Design review of the part built by this model. Coordinates are the model's own, in mm. A direction names the side the tool comes from. Give positions to 0.01 mm unless a question says otherwise; leave off trailing zeros. Loops run counter-clockwise (first coordinate to the right, second up) from the corner with the lowest first, then second, coordinate; pieces in that order, holes last. Notation, with made-up numbers: M -2,6.25 L 55,6.25 A15 ccw 55,13.25 Z; hole C 64,-24.5 d1. An arc over 180 degrees is marked long. Answer as CSV lines item,"result".
```python
from build123d import *

# Parameters (mm, degrees)
SKETCH_1_R          = 5.5
EXTRUDE_1_DEPTH     = 2
SKETCH_2_R          = 3.5
EXTRUDE_2_DEPTH     = 4.5
SKETCH_3_R          = 2
CUT_EXTRUDE_1_DEPTH = 5
CHAMFER_1_SIZE      = 0.5
FILLET_1_R          = 0.2


with BuildPart() as part:
    # 草图1 → 凸台-拉伸1 (new body)
    with BuildSketch(Plane(origin=(0, 0, 0), x_dir=(1, 0, 0), z_dir=(0, 1, 0))):
        with Locations(Location((0, 0, 0), (0, 0, 270))):
            Circle(SKETCH_1_R)
    extrude(amount=EXTRUDE_1_DEPTH)

    # 草图2 → 凸台-拉伸2 (add)
    with BuildSketch(Plane(origin=(0, 2, 0), x_dir=(1, 0, 0), z_dir=(0, 1, 0))):
        with Locations(Location((0, 0, 0), (0, 0, 270))):
            Circle(SKETCH_2_R)
    extrude(amount=EXTRUDE_2_DEPTH)

    # 草图3 → 切除-拉伸1 (cut)
    with BuildSketch(Plane(origin=(0, 6.5, 0), x_dir=(1, 0, 0), z_dir=(0, 1, 0))):
        with Locations(Location((0, 0, 0), (0, 0, 270))):
            Circle(SKETCH_3_R)
    extrude(amount=-CUT_EXTRUDE_1_DEPTH, mode=Mode.SUBTRACT)

    # 倒角1
    chamfer_1_edges = [part.edges().sort_by_distance(p)[0] for p in [
        (0, 0, -5.5),
    ]]
    chamfer(chamfer_1_edges, length=CHAMFER_1_SIZE)

    # 圆角1
    fillet_1_edges = [part.edges().sort_by_distance(p)[0] for p in [
        (0, 6.5, -3.5),
    ]]
    fillet(fillet_1_edges, radius=FILLET_1_R)


solid = part.part
```
1. For P1, Ø3, axis at x = 3, y = 4, coming from the -Z side; P2, Ø2, axis at y = 4, z = 2.5, coming from the -X side; P3, Ø3, axis at x = -3.5, z = 1.5, coming from the +Y side; P4, Ø1.5, axis at x = 3.5, y = 1, coming from the -Z side, all flat-tipped, find the tip position at first contact; note any pin that passes through.
Answer block:
P1,"z = -3.16"
P2,"x = -3.16"
P3,"y = 6.5"
P4,"z = -4.76"
2. We need section A-A, the plane x = 0. Write out the cut boundary in (y, z), plus the area to 3 significant figures.
Answer block:
outline,"M 0,-5 L 0.5,-5.5 L 2,-5.5 L 2,-3.5 L 6.3,-3.5 A0.2 ccw 6.5,-3.3 L 6.5,-2 L 1.5,-2 L 1.5,2 L 6.5,2 L 6.5,3.3 A0.2 ccw 6.3,3.5 L 2,3.5 L 2,5.5 L 0.5,5.5 L 0,5 Z"
area,"33.2 mm²"
3. For faces 4 (the flat face through (0, 2, 4)), 5 (the flat face through (0, 0, 0)), list the 3-axis set-ups (+Z, -Z, +X, -X, +Y, -Y) from which the entire face can be reached by the end or side of a thin tool; tool diameter is ignored.
Answer block:
face 4,"+Y"
face 5,"+Z, -Z, +X, -X, -Y"
4. We need section D-D, the plane y = 1.25. Write out the cut boundary in (x, z), plus the area to 3 significant figures.
Answer block:
outline,"C 0,0 d11"
area,"95.0 mm²"
5. We need section C-C, the plane y = 4.75. Write out the cut boundary in (x, z), plus the area to 3 significant figures.
Answer block:
outline,"C 0,0 d7; hole C 0,0 d4"
area,"25.9 mm²"
6. The part is to be moulded in two halves that separate along Z. For faces 1 (the cylindrical face through (-2, 4, 0)), 2 (the flat face through (-2.2, 6.5, 0)), 3 (the cylindrical face through (-5.37, 1.24, -1.19)), say which applies: pulls with the +Z half, pulls with the -Z half, needs draft (parallel to the pull), parting line crosses it, or undercut.
Answer block:
face 1,"undercut"
face 2,"needs draft"
face 3,"parting line crosses it"
7. We need section B-B, the plane z = 0. Write out the cut boundary in (x, y).
Answer block:
outline,"M -5.5,0.5 L -5,0 L 5,0 L 5.5,0.5 L 5.5,2 L 3.5,2 L 3.5,6.3 A0.2 ccw 3.3,6.5 L 2,6.5 L 2,1.5 L -2,1.5 L -2,6.5 L -3.3,6.5 A0.2 ccw -3.5,6.3 L -3.5,2 L -5.5,2 Z"
8. To check wall thickness, follow L1, parallel to X at y = 5.1, z = 0; L2, parallel to Y at x = -3.75, z = -3; L3, parallel to Z at x = -0.5, y = 6.25. State the ranges of each line that lie inside material, in increasing order. Write a range as [from, to].
Answer block:
L1,"[-3.5, -2], [2, 3.5]"
L2,"[0, 2]"
L3,"[-3.46, -1.94], [1.94, 3.46]"
